Read the model definition and answer for the solid it produces. Units are mm, in the model's axes. Face numbers are marked on the shaded views. A direction names the side the tool comes from. Give positions to 0.01 mm unless a question says otherwise; leave off trailing zeros. Write each loop counter-clockwise with the first axis right and the second up, starting at its lowest first coordinate (ties: lowest second). Pieces come first, ordered by that corner, then holes. Notation, with made-up numbers: (-14, 84) -> (-1, 84) arc R10 ccw to (-1, 101) -> close; hole circle Ø10 at (79, 71.25). An arc over 180 degrees is marked (long way). Use a Markdown table: item, result.
from build123d import *

# Parameters (mm, degrees)
F1_DEPTH = 750


# Not quite as in the source:
# - a pattern or mirror of a feature is missing from the dataset's text; its kind, count and spacing are read off the source's solid


with BuildPart() as f1:
    # F0 (on Front) → F1 (new body)
    with BuildSketch(Plane.XZ):
        Polygon((0, 450), (0, 0), (600, 0), (600, 450), (300, 450), align=None)
        Polygon((0, 850), (0, 450), (300, 450), (150, 850), align=None)
    extrude(amount=F1_DEPTH)

    # F1_copies: F1 across plane


with BuildPart() as f1_1:
    add(f1.part)
    add(f1.part.mirror(Plane(origin=(0, 0, 0), x_dir=(0, 0, -1), z_dir=(-1, 0, 0))))


solid = f1_1.part
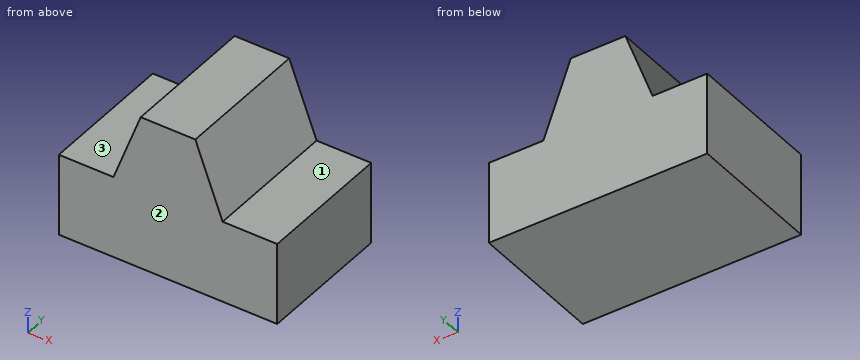
Item 1: Each of these flat-tipped pins is pushed along its axis until it touches: P1, Ø10, axis at y = -256.5, z = 655, coming from the +X side; P2, Ø12, axis at y = -161, z = 631.5, coming from the +X side. Where does it stop, or does it pass through?
Return value:
| item | result |
|---|---|
| P1 | x = 225 |
| P2 | x = 234.19 |
Item 2: A cutting plane is placed at B-B (x = -347). Give the vertices of the cut face in (y, z), then the cut area to 4 significant figures.
Return value:
| item | result |
|---|---|
| outline | (-750, 0) -> (0, 0) -> (0, 450) -> (-750, 450) -> close |
| area | 337,500 mm^2 |
Item 3: A cutting plane is placed at A-A (y = -239.5). Give the vertices of the cut face in (x, z).
Return value:
| item | result |
|---|---|
| outline | (-600, 0) -> (600, 0) -> (600, 450) -> (300, 450) -> (150, 850) -> (-150, 850) -> (-300, 450) -> (-600, 450) -> close |
Item 4: A cutting plane is placed at C-C (z = 479). Give the vertices of the cut face in (x, y) (3 decimals).
Return value:
| item | result |
|---|---|
| outline | (-289.125, -750) -> (289.125, -750) -> (289.125, 0) -> (-289.125, 0) -> close |
Item 5: A tool of negligible diameter and unlimited length cuts with its end or side. For the marked faces 1, 2 and 3, from which of +Z, -Z, +X, -X, +Y, -Y can it reach the whole face along a straight path? Write none if from no direction.
Return value:
| item | result |
|---|---|
| face 1 | +Z, +X, +Y, -Y |
| face 2 | +Z, -Z, +X, -X, -Y |
| face 3 | +Z, -X, +Y, -Y |
Item 6: Straight lines are drawn through the part: line 1 along Z through (x, y) = (-449, -344); line 2 along X through (y, z) = (-265, 533) (3 decimals); line 3 along X through (y, z) = (-106.5, 646). For each, find the intervals that lie inside material, in ascending order. Write a range as [from, to].
Return value:
| item | result |
|---|---|
| line 1 | [0, 450] |
| line 2 | [-268.875, 268.875] |
| line 3 | [-226.5, 226.5] |
